The figure shows three views and two pictorial views of one solid part (mm, origin at its lowest corner). Answer the questions. Give positions to 0.01 mm unless a question says otherwise; leave off trailing zeros. Write each loop counter-clockwise with the first axis right and the second up, starting at its lowest first coordinate (ties: lowest second). Pieces come first, ordered by that corner, then holes. Notation, with made-up numbers: (48.5, 76) - (83.5, 76) arc R24 ccw to (83.5, 95) - close; hole circle Ø8 at (18, -9). An arc over 180 degrees is marked (long way). One line per question, with ' | ' between items. Start each with the question number.
1. The mould has two halves that part along Y. Classify the marked faces 1, 2, 3 and 4: +Y half, -Y half, draft (parallel to the pull), parting line (faces both ways), or undercut.
2. A cutting plane is placed at A-A (z = 4.2). Determine the outline of the cut face in (x, y) (1 decimal).
3. A cutting plane is placed at B-B (y = 7.5). Determine the outline of the cut face in (x, z).
4. Given P1, Ø1.5, axis at x = 2.5, z = 3, coming from the -Y side; P2, Ø1.5, axis at y = 4.5, z = 4, coming from the +X side; P3, Ø2, axis at y = 2.5, z = 1.5, coming from the -X side, each flat-ended and moving along its own axis, determine where each tip first touches the part or whether it passes through.
5. Find the intervals of material crossed by L1, parallel to X at y = 8.25, z = 3.6; L2, parallel to X at y = 12.75, z = 1.9, in increasing order. Write a range as from..to.
6. A cutting plane is placed at D-D (y = 1.5). Determine the outline of the cut face in (x, z), then the cut area to 3 significant figures.
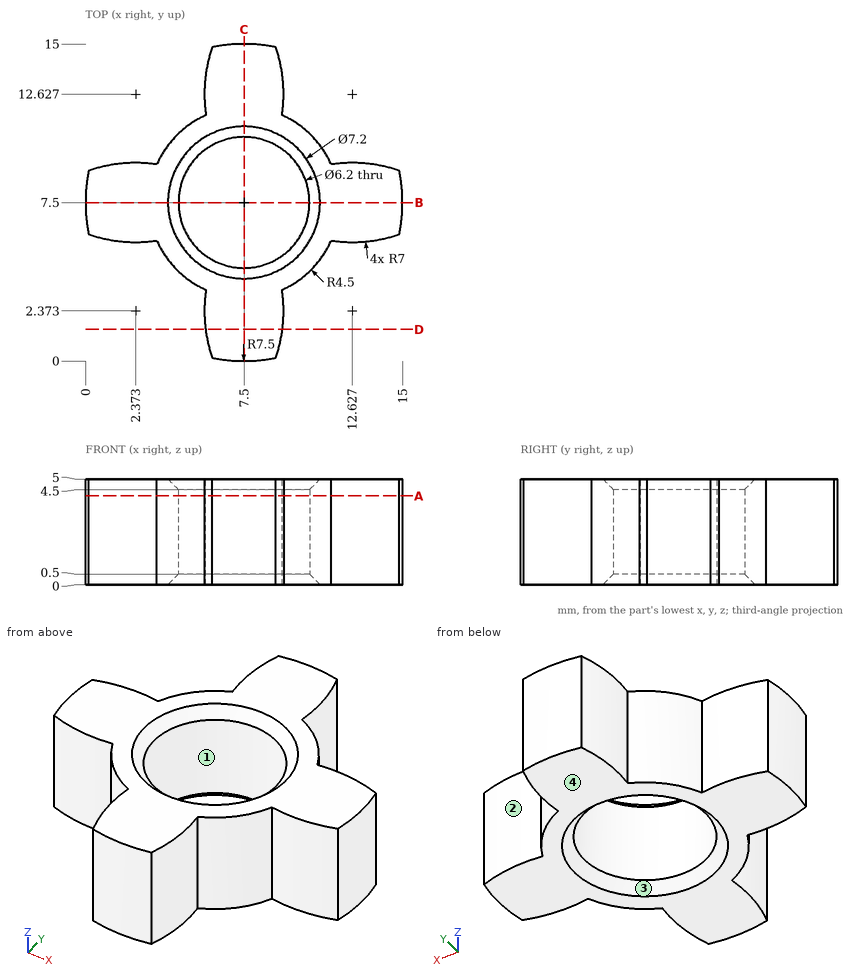
Determined:
1) face 1: undercut | face 2: +Y half | face 3: undercut | face 4: draft
2) outline: (0.2, 6) arc R7 ccw to (3.4, 5.7) arc R4.5 ccw to (5.7, 3.4) arc R7 ccw to (6, 0.2) arc R7.5 ccw to (9, 0.2) arc R7 ccw to (9.3, 3.4) arc R4.5 ccw to (11.6, 5.7) arc R7 ccw to (14.8, 6) arc R7.5 ccw to (14.8, 9) arc R7 ccw to (11.6, 9.3) arc R4.5 ccw to (9.3, 11.6) arc R7 ccw to (9, 14.8) arc R7.5 ccw to (6, 14.8) arc R7 ccw to (5.7, 11.6) arc R4.5 ccw to (3.4, 9.3) arc R7 ccw to (0.2, 9) arc R7.5 ccw to start; hole circle Ø6.2 at (7.5, 7.5)
3) outline: (0, 0) - (3.9, 0) - (4.4, 0.5) - (4.4, 4.5) - (3.9, 5) - (0, 5) - close; (10.6, 0.5) - (11.1, 0) - (15, 0) - (15, 5) - (11.1, 5) - (10.6, 4.5) - close
4) P1: y = 5.63 | P2: x = 11.4 | P3: x = 5.44
5) L1: 0.04..4.49, 10.51..14.96 | L2: 5.63..9.37
6) outline: (5.68, 0) - (9.32, 0) - (9.32, 5) - (5.68, 5) - close | area: 18.2 mm2
